```python
from build123d import *

# Parameters (mm, degrees)
F2_R     = 2.5
F3_DEPTH = 23.001
F4_R     = 5
F4_R_2   = 2.5
F5_DEPTH = 6.5
F6_W     = 137.496356
F6_H     = 90.131391
F7_DEPTH = 57.001


with BuildPart() as f1:
    # F0 (on Front) → F1 (revolve)
    with BuildSketch(Plane.XZ):
        with BuildLine():
            Line((19, 21.923511), (5, 21.923511))
            Line((5, 21.923511), (5, 16.923511))
            Line((5, 16.923511), (-15, 16.923511))
            Line((-15, 16.923511), (-15, 6.923511))
            Line((-15, 6.923511), (4, 6.923511))
            Line((4, 6.923511), (4, 2.12446))
            ThreePointArc((4, 2.12446), (4.679018, 1.859872), (5, 1.205621))
            Line((5, 1.205621), (5, -6.076489))
            Line((5, -6.076489), (8.5, -6.076489))
            Line((8.5, -6.076489), (8.5, -3.076489))
            Line((8.5, -3.076489), (20, -3.076489))
            Line((20, -3.076489), (20, 11.923511))
            Line((20, 11.923511), (18, 11.923511))
            Line((18, 11.923511), (18, 13.923511))
            Line((18, 13.923511), (20, 13.923511))
            Line((20, 13.923511), (20, 15.923511))
            Line((20, 15.923511), (19, 15.923511))
            Line((19, 15.923511), (19, 21.923511))
        make_face()
    revolve(axis=Axis((42, 0, 16.450874), (0, 0, -1)))

    # F2 (on face) → F3 (cut, through all)
    with BuildSketch(Plane.XY.offset(16.923511)):
        with Locations((-1, 0)):
            Circle(F2_R)
        with Locations((85, 0)):
            Circle(F2_R)
        with Locations((42, 43)):
            Circle(F2_R)
        with Locations((42, -43)):
            Circle(F2_R)
    extrude(amount=-F3_DEPTH, mode=Mode.SUBTRACT)

    # F4 (on face) → F5 (cut)
    with BuildSketch(Plane.XY.offset(16.923511)):
        with Locations((-1, 0)):
            Circle(F4_R)
        with Locations((-1, 0)):
            Circle(F4_R_2, mode=Mode.SUBTRACT)
        with Locations((42, 43)):
            Circle(F4_R)
        with Locations((42, 43)):
            Circle(F4_R_2, mode=Mode.SUBTRACT)
        with Locations((85, 0)):
            Circle(F4_R)
        with Locations((85, 0)):
            Circle(F4_R_2, mode=Mode.SUBTRACT)
        with Locations((42, -43)):
            Circle(F4_R)
        with Locations((42, -43)):
            Circle(F4_R_2, mode=Mode.SUBTRACT)
    extrude(amount=-F5_DEPTH, mode=Mode.SUBTRACT)

    # F6 (on Front) → F7 (cut, through all)
    with BuildSketch(Plane.XZ):
        with Locations((31.107662, 6.20803)):
            Rectangle(F6_W, F6_H)
    extrude(amount=-F7_DEPTH, mode=Mode.SUBTRACT)


solid = f1.part
```
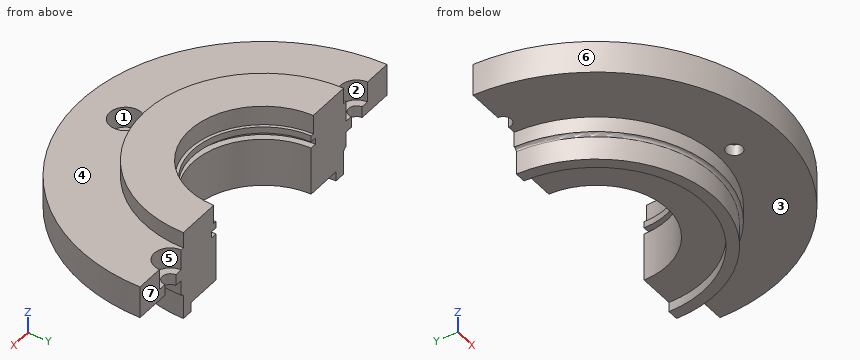
Can you work these out from the model? Positions are in its coordinate system, mm. Face numbers are marked on the shaded views. A direction names the side the tool comes from. Coordinates: 2 decimals unless noted, no trailing zeros. Loops run counter-clockwise (first coordinate to the right, second up) from the corner with the lowest first, then second, coordinate; pieces in that order, holes last. Notation, with made-up numbers: M 51,-3.75 L 72,-3.75 A9 cw 72,9.25 Z; hole C 62.25,20 d7. An arc over 180 degrees is marked long. Put each result on its own line as item: value. Start each with the question number.
(1) Imagine slicing it at A-A on x = 42. List the corners of the cut face in (y, z) for me.
(2) Which directions (+Z, -Z, +X, -X, +Y, -Y) give clear straight access to the entire face, cutting with the end or side of a thin tool? Please do the marked faces 1, 2, 3 and 4.
(3) I need wall thicknesses on probe 1 along Y at (x, z) = (42, 12.5); probe 2 along Y at (x, z) = (42, 9.6); probe 3 along Z at (x, y) = (31, -25.5). Which ranges of each line are inside material? Lowest first, please.
(4) Imagine slicing it at B-B on z = 5.75. List the corners of the cut face in (x, y) for me, and give its area (3 significant figures).
(5) Imagine slicing it at C-C on x = 85. List the corners of the cut face in (y, z) for me, and give its area (3 significant figures).
(6) Will these pins go through, and if not, where does the flat tip stop? pin 1 Ø10 at (y, z) = (-50, 11.5) entering from +X; pin 2 Ø1 at (y, z) = (-46.5, 19) entering from -X; pin 3 Ø11 at (x, y) = (42, -44.5) entering from +Z; pin 4 Ø17 at (x, y) = (31.5, -19.5) entering from -Z.
(7) We'd pull the mould along X, two halves only. Please class the marked faces 5, 6 and 7: +X half, -X half, draft (parallel to the pull), parting line (faces both ways), or undercut.
(8) Imagine slicing it at D-D on y = -53. List the corners of the cut face in (x, z) for me.
Worked answers:
1. outline: M -57,6.92 L -45.5,6.92 L -45.5,10.42 L -48,10.42 L -48,16.92 L -57,16.92 Z; M -40.5,6.92 L -38,6.92 L -38,2.12 A1 cw -37,1.21 L -37,-6.08 L -33.5,-6.08 L -33.5,-3.08 L -22,-3.08 L -22,11.92 L -24,11.92 L -24,13.92 L -22,13.92 L -22,15.92 L -23,15.92 L -23,21.92 L -37,21.92 L -37,16.92 L -38,16.92 L -38,10.42 L -40.5,10.42 Z
2. face 1: +Z
2. face 2: +Z, +Y
2. face 3: -Z, -Y
2. face 4: +Z, -Y
3. probe 1: y = -57 to -48, -38 to -24
3. probe 2: y = -57 to -45.5, -40.5 to -22
3. probe 3: z = -3.08 to 21.92
4. outline: M 4,0 A38 ccw 80,0 L 64,0 A22 cw 20,0 Z
4. area: 1,510 mm2
5. outline: M -37.42,6.92 L -2.5,6.92 L -2.5,10.42 L -5,10.42 L -5,16.92 L -37.42,16.92 Z
5. area: 333 mm2
6. pin 1: stops at x = 76.99
6. pin 2: passes through
6. pin 3: stops at z = 16.92
6. pin 4: stops at z = -3.08
7. face 5: undercut
7. face 6: parting line
7. face 7: draft
8. outline: M 21.02,6.92 L 62.98,6.92 L 62.98,16.92 L 21.02,16.92 Z
